Design review of the part built by this model. Coordinates are the model's own, in mm. A direction names the side the tool comes from. Give positions to 0.01 mm unless a question says otherwise; leave off trailing zeros. Write each loop counter-clockwise with the first axis right and the second up, starting at its lowest first coordinate (ties: lowest second). Pieces come first, ordered by that corner, then holes. Notation, with made-up numbers: M 67,-6 L 107,-6 A12 cw 107,16 Z; hole C -3,70.5 d4. An arc over 180 degrees is marked long. Answer in a Markdown table with one row per item.
```python
from build123d import *

# Parameters (mm, degrees)
SKETCH1_R           = 50
SKETCH1_R_2         = 1.9
BOSS_EXTRUDE1_DEPTH = 12
CUT_EXTRUDE5_DEPTH  = 12
SKETCH8_R           = 1.5
CUT_EXTRUDE8_DEPTH  = 10


with BuildPart() as part:
    # Sketch1 → Boss-Extrude1 (new body)
    with BuildSketch(Plane(origin=(0, 0, 0), x_dir=(1, 0, 0), z_dir=(0, 1, 0))):
        with Locations(Location((0, 0, 0), (0, 0, 270))):
            Circle(SKETCH1_R)
        with Locations(Location((0, 0, 0), (0, 0, 270))):
            Circle(SKETCH1_R_2, mode=Mode.SUBTRACT)
    extrude(amount=BOSS_EXTRUDE1_DEPTH)

    # Sketch3 → Cut-Extrude5 (cut)
    with BuildSketch(Plane(origin=(0, 12, 0), x_dir=(1, 0, 0), z_dir=(0, 1, 0))):
        with BuildLine():
            ThreePointArc((-4.207984423, -10.16330985), (-9.0163955, -9.369996887), (-13.679908421, -10.784850156))
            Line((-13.679908421, -10.784850156), (-29.375319677, -19.846600069))
            ThreePointArc((-29.375319677, -19.846600069), (-31.335687043, -22.658660307), (-30.427937323, -25.964218268))
            ThreePointArc((-30.427937323, -25.964218268), (0, -40), (30.427937323, -25.964218268))
            ThreePointArc((30.427937323, -25.964218268), (31.335687043, -22.658660307), (29.375319677, -19.846600069))
            Line((29.375319677, -19.846600069), (13.679908421, -10.784850156))
            ThreePointArc((13.679908421, -10.784850156), (9.0163955, -9.369996887), (4.207984423, -10.16330985))
            ThreePointArc((4.207984423, -10.16330985), (0, -11), (-4.207984423, -10.16330985))
        make_face()
        with BuildLine():
            ThreePointArc((-6.697692305, 8.725876334), (-3.606457588, 12.493425997), (-2.5, 17.239573292))
            Line((-2.5, 17.239573292), (-2.5, 35.363073119))
            ThreePointArc((-2.5, 35.363073119), (-3.95513192, 38.466831178), (-7.271703949, 39.33347584))
            ThreePointArc((-7.271703949, 39.33347584), (-34.641016151, 20), (-37.699641271, -13.369257572))
            ThreePointArc((-37.699641271, -13.369257572), (-35.290818963, -15.808170871), (-31.875319677, -15.51647305))
            Line((-31.875319677, -15.51647305), (-16.179908421, -6.454723137))
            ThreePointArc((-16.179908421, -6.454723137), (-12.622853088, -3.12342911), (-10.905676728, 1.437433516))
            ThreePointArc((-10.905676728, 1.437433516), (-9.526279442, 5.5), (-6.697692305, 8.725876334))
        make_face()
        with BuildLine():
            Line((2.5, 35.363073119), (2.5, 17.239573292))
            ThreePointArc((2.5, 17.239573292), (3.606457588, 12.493425997), (6.697692305, 8.725876334))
            ThreePointArc((6.697692305, 8.725876334), (9.526279442, 5.5), (10.905676728, 1.437433516))
            ThreePointArc((10.905676728, 1.437433516), (12.622853088, -3.12342911), (16.179908421, -6.454723137))
            Line((16.179908421, -6.454723137), (31.875319677, -15.51647305))
            ThreePointArc((31.875319677, -15.51647305), (35.290818963, -15.808170871), (37.699641271, -13.369257572))
            ThreePointArc((37.699641271, -13.369257572), (39.420715689, -6.782858879), (40, 0))
            ThreePointArc((40, 0), (30.747911782, 25.584485944), (7.271703949, 39.33347584))
            ThreePointArc((7.271703949, 39.33347584), (3.95513192, 38.466831178), (2.5, 35.363073119))
        make_face()
    extrude(amount=-CUT_EXTRUDE5_DEPTH, mode=Mode.SUBTRACT)

    # Sketch7 → Cut-Revolve1 (revolve, cut)
    with BuildSketch(Plane.XY):
        Polygon((40, 12), (30.939044017, 5), (0, 5), (0, 12), align=None)
    revolve(axis=Axis((0, 5, 0), (0, 1, 0)), mode=Mode.SUBTRACT)

    # Sketch8 → Cut-Extrude8 (cut)
    with BuildSketch(Plane(origin=(0, 0, 0), x_dir=(1, 0, 0), z_dir=(0, 1, 0))):
        with Locations((0, 8)):
            Circle(SKETCH8_R)
        with Locations((8, 0)):
            Circle(SKETCH8_R)
        with Locations((0, -8)):
            Circle(SKETCH8_R)
        with Locations((-8, 0)):
            Circle(SKETCH8_R)
    extrude(amount=CUT_EXTRUDE8_DEPTH, mode=Mode.SUBTRACT)


solid = part.part
```
1) Insertion check: P1, Ø2.5, axis at y = 4.5, z = -24.5, coming from the -X side; P2, Ø5, axis at y = 6, z = -7.5, coming from the +X side; P3, Ø6, axis at x = -11, y = 5, coming from the +Z side. Each pin has a flat end and moves straight along its axis. Give the tip position at first contact, or say it passes through.
Geometry says:
| item | result |
|---|---|
| P1 | x = -44.27 |
| P2 | x = 49.75 |
| P3 | z = 49.36 |
2) Add section D-D (z = 37.5). Write out the cut boundary in (x, y).
Geometry says:
| item | result |
|---|---|
| outline | M -33.07,0 L -13.92,0 L -13.92,12 L -33.07,12 Z; M 13.92,0 L 33.07,0 L 33.07,12 L 13.92,12 Z |
3) Add section C-C (y = 3). Count the separate pieces of the cut face and the enclosed holes in it, and give its area (3 significant figures).
Geometry says:
| item | result |
|---|---|
| separate pieces | 1 |
| enclosed holes | 8 |
| area | 3,670 mm^2 |
4) The part is to be moulded in two halves that separate along X. For faces 3 (the face through (2.5, 2, -26)), 4 (the face through (15.02, 5.92, 47.69)), say which applies: released by +X, released by -X, zero draft, split by the parting line, or undercut.
Geometry says:
| item | result |
|---|---|
| face 3 | undercut |
| face 4 | split by the parting line |
5) Add section A-A (x = 0). Write out the cut boundary in (y, z), and give its area (3 significant figures).
Geometry says:
| item | result |
|---|---|
| outline | M 0,-50 L 12,-50 L 12,-40 L 5,-30.94 L 5,-9.5 L 0,-9.5 Z; M 0,-6.5 L 5,-6.5 L 5,-1.9 L 0,-1.9 Z; M 0,1.9 L 5,1.9 L 5,6.5 L 0,6.5 Z; M 0,9.5 L 5,9.5 L 5,11 L 0,11 Z; M 0,40 L 12,40 L 12,50 L 0,50 Z |
| area | 478 mm^2 |
6) Add section B-B (z = 8). Write out the cut boundary in (x, y).
Geometry says:
| item | result |
|---|---|
| outline | M -49.36,0 L -39.19,0 L -39.19,12 L -49.36,12 Z; M -18.86,0 L -1.5,0 L -1.5,5 L -18.86,5 Z; M 1.5,0 L 18.86,0 L 18.86,5 L 1.5,5 Z; M 39.19,0 L 49.36,0 L 49.36,12 L 39.19,12 Z |
7) For faces 1 (the face through (31.49, 9.23, 18.29)), 2 (the face through (3.993, 6.084, -38.498)), list the 3-axis set-ups (+Z, -Z, +X, -X, +Y, -Y) from which the entire face can be reached by the end or side of a thin tool; tool diameter is ignored.
Geometry says:
| item | result |
|---|---|
| face 1 | +Y |
| face 2 | +Y, -Y |
8) To check wall thickness, follow probe 1 along X at (y, z) = (1.75, 13.5); probe 2 along Z at (x, y) = (-8, 1.7); probe 3 along X at (y, z) = (1.35, 8). State the ranges of each line that lie inside material, in increasing order. Write a range as [from, to].
Geometry says:
| item | result |
|---|---|
| probe 1 | [-48.14, -37.65], [-28.38, -18.38], [18.38, 28.38], [37.65, 48.14] |
| probe 2 | [-49.36, -39.19], [-7.55, -1.5], [1.5, 9.35], [39.19, 49.36] |
| probe 3 | [-49.36, -39.19], [-18.86, -1.5], [1.5, 18.86], [39.19, 49.36] |
